Autodesk Inventor part; units mm, degrees
ref_plane "YZ Plane" through (0, 0, 0) normal (1, 0, 0) x (0, 1, 0)
ref_plane "XZ Plane" through (0, 0, 0) normal (0, 1, 0) x (-1, 0, 0)
ref_plane "XY Plane" through (0, 0, 0) normal (0, 0, 1) x (1, 0, 0)
sketch "Sketch2" plane through (0, 0, 0) normal (0, 0, 1) x (1, 0, 0)
  circle A0 centre (0, 0) radius 12.5
  dimension "d0" = 25
extrude "Extrusion1" add sketch "Sketch2" along normal blind 5
sketch "Sketch3" plane through (0, 0, 5) normal (0, 0, 1) x (1, 0, 0)
  line L0 (0, 0) -> (0, 9.5351)
  line L1 (0, 22.5) -> (-4.4873, 11.6668)
  circle A0 centre (0, 0) radius 12.5
  line L2 (0, 22.5) -> (4.4873, 11.6668)
  arc A1 (4.4873, 11.6668) -> (-4.4873, 11.6668) centre (0, 0) ccw
  point P0 (0, 12.5)
  dimension "d3" = 45
  dimension "d4" = 10
extrude "Extrusion2" add sketch "Sketch3" against normal up to surface (5 mm away) contours L2 A0 L1
pattern_circular "Circular Pattern1" count 18 over 360 about axis through (0, 0, 0) along (0, 0, 1) of "Extrusion2"
sketch "Sketch4" plane through (0, 0, 0) normal (0, 0, -1) x (-1, 0, 0)
  point P0 (0, 0)
  point P1 (0, 0)
hole "Hole1" at (0, 0, 0) at (0, 0, 0) direction (0, 0, 1) diameter 4 end through all
properties part number "Drive Gear"
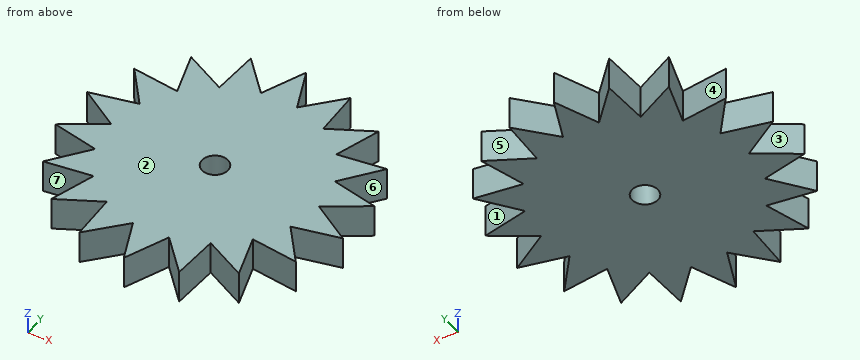
Model file for the job. Use its own axes, mm. Face numbers are marked on the shaded views. A direction names the side the tool comes from. Round coordinates to 2 decimals unless told otherwise and drop trailing zeros. Write each loop counter-clockwise with the first axis right and the second up, starting at its lowest first coordinate (ties: lowest second). Pieces come first, ordered by that corner, then holes. Notation, with made-up numbers: (50, 50.5) - (63, 50.5) arc R19 cw to (63, 76.5) - close; hole circle Ø3 at (77.25, 28). An arc over 180 degrees is marked (long way). One line per item, written item: value.
(1) Cut at A-A, the plane x = 18.5. Give the cut face in (y, z).
Values follow:
outline: (-11.12, 0) - (-9.97, 0) - (-9.97, 5) - (-11.12, 5) - close; (-4.72, 0) - (-1.58, 0) - (-1.58, 5) - (-4.72, 5) - close; (1.58, 0) - (4.72, 0) - (4.72, 5) - (1.58, 5) - close; (9.97, 0) - (11.12, 0) - (11.12, 5) - (9.97, 5) - close
(2) Two-plate mould, pull along X, no slides. Class the marked faces 1, 2, 3 and 4: pulls with the +X half, pulls with the -X half, needs draft (parallel to the pull), parting line crosses it, or undercut.
Values follow:
face 1: pulls with the +X half
face 2: needs draft
face 3: pulls with the -X half
face 4: undercut
(3) Wall check: probe 1 along Y at (x, z) = (-16.5, 4.35); probe 2 along X at (y, z) = (-16, 0.7); probe 3 along X at (y, z) = (1.5, 4.55). Give the ranges that are in metal, low to high.
Values follow:
probe 1: y = -10.86 to -7.36, -5.16 to -0.3, 0.3 to 5.16, 7.36 to 10.86
probe 2: x = -14.07 to -12.09, -7.92 to -2.98, -2.69 to 2.69, 2.98 to 7.92, 12.09 to 14.07
probe 3: x = -18.38 to -1.32, 1.32 to 18.38
(4) Drop flat-ended pins along their axis: P1, Ø3, axis at x = -17.5, z = 2, coming from the -Y side; P2, Ø2, axis at y = -11, z = 1.5, coming from the +X side. Give the stop position or say it passes through.
Values follow:
P1: stops at y = -11.19
P2: stops at x = 19.49
(5) Cut at B-B, the plane x = 7. Give the cut face in (y, z).
Values follow:
outline: (-20.38, 0) - (20.38, 0) - (20.38, 5) - (-20.38, 5) - close
(6) 3-axis set-ups, long thin cutter, end or side, ignore diameter. For the marked faces 5, 6 and 7: which of +Z, -Z, +X, -X, +Y, -Y reach the whole face in a straight line?
Values follow:
face 5: +Z, -Z, +Y
face 6: +Z, -Z, +X
face 7: +Z, -Z
